Verification items for the finished model (mm, model axes). Give positions to 0.01 mm unless a question says otherwise; leave off trailing zeros. Write each loop counter-clockwise with the first axis right and the second up, starting at its lowest first coordinate (ties: lowest second). Pieces come first, ordered by that corner, then holes.
from build123d import *

# Parameters (mm, degrees)
SKETCH1_W           = 416
SKETCH1_H           = 106
BOSS_EXTRUDE1_DEPTH = 3
SKETCH2_W           = 3
SKETCH2_H           = 14
SKETCH2_W_2         = 14
SKETCH2_H_2         = 3
CUT_EXTRUDE1_DEPTH  = 3
CUT_EXTRUDE2_DEPTH  = 3


with BuildPart() as part:
    # Sketch1 → Boss-Extrude1 (new body)
    with BuildSketch(Plane.XY):
        with Locations((0, -3)):
            Rectangle(SKETCH1_W, SKETCH1_H)
    extrude(amount=BOSS_EXTRUDE1_DEPTH)

    # Sketch2 → Cut-Extrude1 (cut)
    with BuildSketch(Plane.XY.offset(3)):
        with Locations((201.5, 26)):
            Rectangle(SKETCH2_W, SKETCH2_H)
        with Locations((-201.5, 26)):
            Rectangle(SKETCH2_W, SKETCH2_H)
        with Locations((201.5, -26)):
            Rectangle(SKETCH2_W, SKETCH2_H)
        with Locations((-201.5, -26)):
            Rectangle(SKETCH2_W, SKETCH2_H)
        with Locations((174, -51.5)):
            Rectangle(SKETCH2_W_2, SKETCH2_H_2)
        with Locations((-174, -51.5)):
            Rectangle(SKETCH2_W_2, SKETCH2_H_2)
        with Locations((58, -51.5)):
            Rectangle(SKETCH2_W_2, SKETCH2_H_2)
        with Locations((-58, -51.5)):
            Rectangle(SKETCH2_W_2, SKETCH2_H_2)
    extrude(amount=-CUT_EXTRUDE1_DEPTH, mode=Mode.SUBTRACT)

    # Sketch4 → Cut-Extrude2 (cut)
    with BuildSketch(Plane.XY.offset(3)):
        with BuildLine():
            Line((-175, -5), (-85, -5))
            ThreePointArc((-85, -5), (-65, -25), (-85, -45))
            Line((-85, -45), (-175, -45))
            ThreePointArc((-175, -45), (-195, -25), (-175, -5))
        make_face()
    extrude(amount=-CUT_EXTRUDE2_DEPTH, mode=Mode.SUBTRACT)


solid = part.part
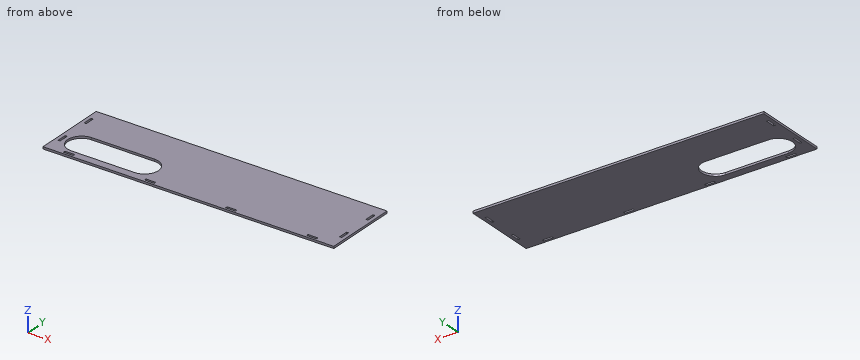
Item 1: Sectioned sample at A-A on y = -25. Record the cut outline in (x, z).
Answer key:
outline: (-208, 0) - (-203, 0) - (-203, 3) - (-208, 3) - close; (-200, 0) - (-195, 0) - (-195, 3) - (-200, 3) - close; (-65, 0) - (200, 0) - (200, 3) - (-65, 3) - close; (203, 0) - (208, 0) - (208, 3) - (203, 3) - close
Item 2: Scan lines: line 1 along X through (y, z) = (32.5, 2.35); line 2 along X through (y, z) = (-24.5, 1.05); line 3 along X through (y, z) = (-40.5, 2.7). Record each from-to range of solid material in increasing order.
Answer key:
line 1: x = -208 to -203, -200 to 200, 203 to 208
line 2: x = -208 to -203, -200 to -194.99, -65.01 to 200, 203 to 208
line 3: x = -208 to -187.64, -72.36 to 208
Item 3: Sectioned sample at B-B on x = 174.5. Record the cut outline in (y, z).
Answer key:
outline: (-56, 0) - (-53, 0) - (-53, 3) - (-56, 3) - close; (-50, 0) - (50, 0) - (50, 3) - (-50, 3) - close
Item 4: Sectioned sample at C-C on z = 2.3. State how many separate pieces and enclosed holes the cut face has, then the cut area to 3 significant figures.
Answer key:
separate pieces: 1
enclosed holes: 9
area: 38,900 mm2
